Read the model definition and answer for the solid it produces. Units are mm, in the model's axes. Face numbers are marked on the shaded views. A direction names the side the tool comes from. Coordinates: 2 decimals unless noted, no trailing zeros. Loops run counter-clockwise (first coordinate to the right, second up) from the corner with the lowest first, then second, coordinate; pieces in that order, holes last.
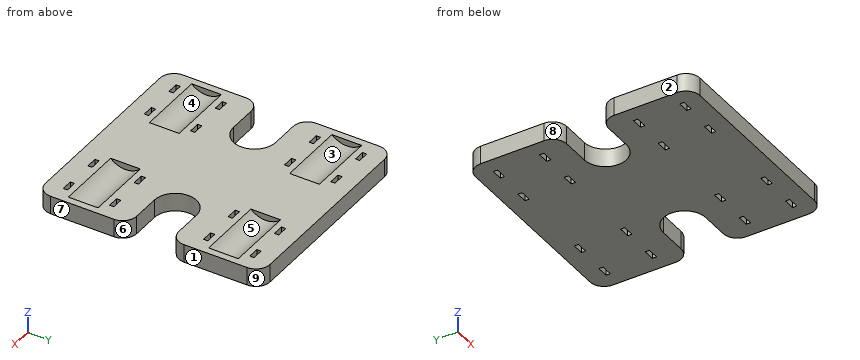
Autodesk Inventor part; units mm, degrees
ref_plane "YZ Plane" through (0, 0, 0) normal (1, 0, 0) x (0, 1, 0)
ref_plane "XZ Plane" through (0, 0, 0) normal (0, 1, 0) x (-1, 0, 0)
ref_plane "XY Plane" through (0, 0, 0) normal (0, 0, 1) x (1, 0, 0)
sketch "Sketch1" plane through (0, 0, 0) normal (0, 0, 1) x (1, 0, 0)
  line L0 (-37.5, 40) -> (37.5, 40)
  line L1 (37.5, 40) -> (37.5, -40)
  line L2 (37.5, -40) -> (-37.5, -40)
  line L3 (-37.5, -40) -> (-37.5, 40)
  point P0 (0, 0)
  point P1 (37.5, 0)
  point P2 (0, 40)
  dimension "d0" = 75
  dimension "d2" = 80
extrude "Extrusion1" add sketch "Sketch1" along normal blind 6.477
sketch "Sketch2" plane through (0, 0, 6.477) normal (0, 0, 1) x (1, 0, 0)
  line L0 (-37.5, 40) -> (-37.5, -40)
  line L1 (-11, 19.6967) -> (11, 19.6967) construction
  line L2 (11, 19.6967) -> (11, -19.6967) construction
  line L3 (11, -19.6967) -> (-11, -19.6967) construction
  line L4 (-11, -19.6967) -> (-11, 19.6967) construction
  line L5 (-11, 19.6967) -> (-35, 19.6967)
  line L6 (-35, 19.6967) -> (-35, 30.3033)
  line L7 (-35, 30.3033) -> (-11, 30.3033)
  line L8 (-11, 30.3033) -> (-11, 19.6967)
  line L9 (11, 19.6967) -> (35, 19.6967)
  line L10 (35, 19.6967) -> (35, 30.3033)
  line L11 (35, 30.3033) -> (11, 30.3033)
  line L12 (11, 30.3033) -> (11, 19.6967)
  line L13 (-11, -19.6967) -> (-35, -19.6967)
  line L14 (-35, -19.6967) -> (-35, -30.3033)
  line L15 (-35, -30.3033) -> (-11, -30.3033)
  line L16 (-11, -30.3033) -> (-11, -19.6967)
  line L17 (11, -19.6967) -> (35, -19.6967)
  line L18 (35, -19.6967) -> (35, -30.3033)
  line L19 (35, -30.3033) -> (11, -30.3033)
  line L20 (11, -30.3033) -> (11, -19.6967)
  circle A0 centre (-11, 25) radius 7.5 construction
  line L21 (-11, 25) -> (-5.6967, 19.6967) construction
  point P0 (0, 0)
  point P1 (-11, 0)
  point P2 (0, 19.6967)
  dimension "d11" = 15
  dimension "d5" = 50
  dimension "d7" = 24
  dimension "d9" = 2.5
  dimension "d10" = 45
extrude "Extrusion2" cut sketch "Sketch2" against normal through all
sketch "Sketch3" plane through (-35, 19.6967, 6.477) normal (1, 0, 0) x (0, 0, -1)
  line L0 (6.477, 10.6066) -> (6.477, 0)
  line L1 (0, 10.6066) -> (6.477, 10.6066)
  line L2 (0, 0) -> (0, 10.6066)
  line L3 (0, 0) -> (6.477, 0)
  line L4 (6.477, -39.3934) -> (6.477, -50)
  line L5 (0, -39.3934) -> (6.477, -39.3934)
  line L6 (0, -50) -> (0, -39.3934)
  line L7 (0, -50) -> (6.477, -50)
  arc A0 (0, 0) -> (0, 10.6066) centre (-5.3033, 5.3033) ccw
  arc A1 (0, -50) -> (0, -39.3934) centre (-5.3033, -44.6967) ccw
  point P0 (6.477, -19.6967)
  dimension "d14" = 15
extrude "Extrusion3" add sketch "Sketch3" along normal up to surface (70 mm away) contours L0 L3 A0 L1 | L4 L7 A1 L5
sketch "Sketch4" plane through (0, 0, 6.477) normal (0, 0, 1) x (1, 0, 0)
  line L0 (-35, 19.6967) -> (-35, 30.3033)
  line L1 (-35, 30.3033) -> (-11, 30.3033)
  line L2 (-11, 30.3033) -> (-11, 19.6967)
  line L3 (-28, 32.5) -> (-18, 32.5) construction
  line L4 (-18, 32.5) -> (-18, 17.5) construction
  line L5 (-18, 17.5) -> (-28, 17.5) construction
  line L6 (-28, 17.5) -> (-28, 32.5) construction
  line L7 (-28, 32.5) -> (-32, 32.5)
  line L8 (-32, 32.5) -> (-32, 34)
  line L9 (-32, 34) -> (-28, 34)
  line L10 (-28, 34) -> (-28, 32.5)
  line L11 (-18, 32.5) -> (-14, 32.5)
  line L12 (-14, 32.5) -> (-14, 34)
  line L13 (-14, 34) -> (-18, 34)
  line L14 (-18, 34) -> (-18, 32.5)
  line L15 (-18, 17.5) -> (-14, 17.5)
  line L16 (-14, 17.5) -> (-14, 16)
  line L17 (-14, 16) -> (-18, 16)
  line L18 (-18, 16) -> (-18, 17.5)
  line L19 (-28, 17.5) -> (-32, 17.5)
  line L20 (-32, 17.5) -> (-32, 16)
  line L21 (-32, 16) -> (-28, 16)
  line L22 (-28, 16) -> (-28, 17.5)
  point P0 (0, 0)
  point P1 (-23, 32.5)
  point P2 (-23, 30.3033)
  point P3 (-18, 25)
  point P4 (-11, 25)
  point P5 (-30, 34)
  dimension "d18" = 5
  dimension "d19" = 15
  dimension "d20" = 4
  dimension "d21" = 1.5
extrude "Extrusion4" cut sketch "Sketch4" against normal through all
mirror "Mirror1" about plane through (0, 0, 0) normal (1, 0, 0) of "Extrusion4"
mirror "Mirror2" about plane through (0, 0, 0) normal (0, 1, 0) of "Extrusion4", "Mirror1"
fillet "Fillet1" radius 5 4 edges at (-37.5, 40, 3.2385) (-37.5, -40, 3.2385) (37.5, -40, 3.2385) (37.5, 40, 3.2385)
sketch "Sketch6" plane through (0, 0, 6.477) normal (0, 0, 1) x (1, 0, 0)
  line L0 (-37.5, 35) -> (-37.5, -35)
  line L1 (37.5, -35) -> (37.5, 35)
  line L2 (-11, -19.6967) -> (-11, -30.3033)
  line L3 (-37.5, 7.5) -> (-22.5, 7.5)
  arc A0 (-22.5, -7.5) -> (-22.5, 7.5) centre (-22.5, 0) ccw
  line L4 (-22.5, -7.5) -> (-37.5, -7.5)
  line L5 (37.5, -7.5) -> (22.5, -7.5)
  arc A1 (22.5, 7.5) -> (22.5, -7.5) centre (22.5, 0) ccw
  line L6 (22.5, 7.5) -> (37.5, 7.5)
  point P0 (0, 0)
  dimension "d31" = 7.5
  dimension "d33" = 15
extrude "Extrusion6" cut sketch "Sketch6" against normal through all
fillet "Fillet3" radius 5 4 edges at (-37.5, -7.5, 3.2385) (-37.5, 7.5, 3.2385) (37.5, 7.5, 3.2385) (37.5, -7.5, 3.2385)
properties part number "EFFECTOR BEARING PLATE"
Item 1: A cutting plane is placed at A-A on x = -29.5. Determine the outline of the cut face in (y, z), then the cut area to 3 significant figures.
Numbers:
outline: (-40, 0) - (-34, 0) - (-34, 6.48) - (-40, 6.48) - close; (-32.5, 0) - (-17.5, 0) - (-17.5, 6.48) - (-19.7, 6.48) arc R7.5 cw to (-30.3, 6.48) - (-32.5, 6.48) - close; (-16, 0) - (-7.5, 0) - (-7.5, 6.48) - (-16, 6.48) - close; (7.5, 0) - (16, 0) - (16, 6.48) - (7.5, 6.48) - close; (17.5, 0) - (32.5, 0) - (32.5, 6.48) - (30.3, 6.48) arc R7.5 cw to (19.7, 6.48) - (17.5, 6.48) - close; (34, 0) - (40, 0) - (40, 6.48) - (34, 6.48) - close
area: 350 mm2
Item 2: A cutting plane is placed at C-C on y = -23. Determine the outline of the cut face in (x, z).
Numbers:
outline: (-37.5, 0) - (37.5, 0) - (37.5, 6.48) - (35, 6.48) - (35, 4.55) - (11, 4.55) - (11, 6.48) - (-11, 6.48) - (-11, 4.55) - (-35, 4.55) - (-35, 6.48) - (-37.5, 6.48) - close
Item 3: A cutting plane is placed at D-D on y = 0. Determine the outline of the cut face in (x, z), then the cut area to 3 significant figures.
Numbers:
outline: (-15, 0) - (15, 0) - (15, 6.48) - (-15, 6.48) - close
area: 194 mm2
Item 4: Which of the six approach directions +Z, -Z, +X, -X, +Y, -Y give full straight-line access (tool end or side, diameter ignored) to the marked faces 5, 6, 7, 8 and 9?
Numbers:
face 5: +Z
face 6: +Z, -Z, +X
face 7: +Z, -Z, +X, +Y, -Y
face 8: +Z, -Z, -X
face 9: +Z, -Z, +X, +Y
Item 5: Determine the mould class of the marked faces 1, 2, 3 and 4 for opening direction X: released by +X, released by -X, zero draft, split by the parting line, or undercut.
Numbers:
face 1: released by +X
face 2: released by -X
face 3: undercut
face 4: undercut
Item 6: Find the intervals of material crossed by line 1 along X through (y, z) = (33, 1.75); line 2 along Y through (x, z) = (-31.5, 0.5); line 3 along Y through (x, z) = (-26, 4), in increasing order.
Numbers:
line 1: x = -37.5 to -32, -28 to -18, -14 to 14, 18 to 28, 32 to 37.5
line 2: y = -40 to -34, -32.5 to -17.5, -16 to -7.5, 7.5 to 16, 17.5 to 32.5, 34 to 40
line 3: y = -40 to -7.5, 7.5 to 40
Item 7: A cutting plane is placed at B-B on y = 29. Determine the outline of the cut face in (x, z), then the cut area to 3 significant figures.
Numbers:
outline: (-37.5, 0) - (37.5, 0) - (37.5, 6.48) - (35, 6.48) - (35, 5.44) - (11, 5.44) - (11, 6.48) - (-11, 6.48) - (-11, 5.44) - (-35, 5.44) - (-35, 6.48) - (-37.5, 6.48) - close
area: 436 mm2
